Check sheet for the drawn part. Datum: minimum x, y, z corner. Units: mm. A direction names the side the tool comes from. Coordinates: 2 decimals unless noted, no trailing zeros. Order: outer loops, then holes, each group sorted by start corner. A loop starts at its lowest first (then second) coordinate and runs counter-clockwise, first axis right, second up. Notation, with made-up numbers: (35, 13) - (67, 13) arc R25 cw to (67, 32) - close; hole circle Ø8 at (81.25, -6). An arc over 180 degrees is marked (long way). Put each result on its own line as item: value.
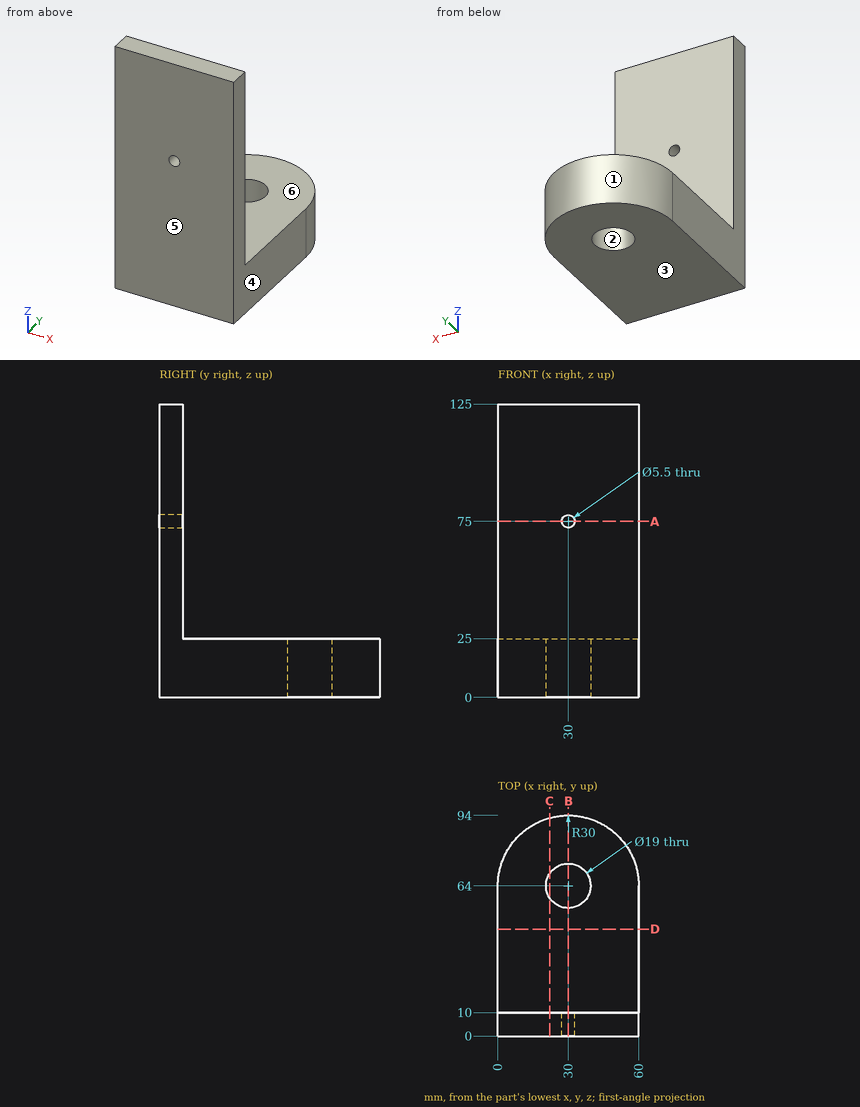
Q1. Section check B-B on x = 30. Record the boundary of the cut face in (y, z).
Answer block:
outline: (0, 0) - (54.5, 0) - (54.5, 25) - (10, 25) - (10, 72.25) - (0, 72.25) - close; (0, 77.75) - (10, 77.75) - (10, 125) - (0, 125) - close; (73.5, 0) - (94, 0) - (94, 25) - (73.5, 25) - close
Q2. Section check D-D on y = 45.5. Record the boundary of the cut face in (x, z), then the cut area to 3 significant figures.
Answer block:
outline: (0, 0) - (60, 0) - (60, 25) - (0, 25) - close
area: 1,500 mm^2
Q3. Access from +Z, -Z, +X, -X, +Y, -Y to the whole of each face (thin tool, end or side, straight path). Record for the marked faces 5 and 6.
Answer block:
face 5: +Z, -Z, +X, -X, -Y
face 6: +Z, +X, -X, +Y
Q4. Depth check by flat-ended pin: pin 1 Ø10 at (x, y) = (46, 33.5) entering from +Z; pin 2 Ø15 at (x, y) = (30, 64) entering from +Z; pin 3 Ø18 at (x, z) = (29, 70.5) entering from +Y; pin 4 Ø10 at (x, z) = (22.5, 27.5) entering from +Y. Enter the tip coordinate at first touch or a pass-through.
Answer block:
pin 1: stops at z = 25
pin 2: passes through
pin 3: stops at y = 10
pin 4: stops at y = 93.83
Q5. Draft check along X on the marked faces 1, 2, 3 and 4. Enter one of: pulls with the +X half, pulls with the -X half, needs draft (parallel to the pull), parting line crosses it, or undercut.
Answer block:
face 1: parting line crosses it
face 2: undercut
face 3: needs draft
face 4: pulls with the +X half
Q6. Section check C-C on x = 22. Record the boundary of the cut face in (y, z), then the cut area to 3 significant figures.
Answer block:
outline: (0, 0) - (58.88, 0) - (58.88, 25) - (10, 25) - (10, 125) - (0, 125) - close; (69.12, 0) - (92.91, 0) - (92.91, 25) - (69.12, 25) - close
area: 3,070 mm^2
Q7. Thickness scan on L1, parallel to Y at x = 30, z = 17; L2, parallel to Y at x = 44, z = 34; L3, parallel to Z at x = 12, y = 46. Record the ranges inside material, lowest first. Write a range as [from, to].
Answer block:
L1: y = [0, 54.5], [73.5, 94]
L2: y = [0, 10]
L3: z = [0, 25]
Q8. Section check A-A on z = 75. Record the boundary of the cut face in (x, y).
Answer block:
outline: (0, 0) - (27.25, 0) - (27.25, 10) - (0, 10) - close; (32.75, 0) - (60, 0) - (60, 10) - (32.75, 10) - close
